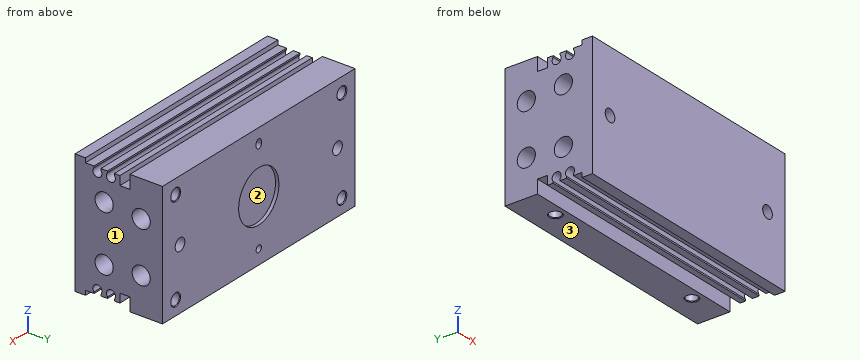
from build123d import *

# Parameters (mm, degrees)
SKETCH2_W                = 55
SKETCH2_H                = 39
BOSS_EXTRUDE1_DEPTH      = 55
CUT_EXTRUDE1_DEPTH       = 65.509689195
CUT_EXTRUDE1_DEPTH_BACK  = 65.509689195
SKETCH3_W                = 2
SKETCH3_H                = 19.8
CUT_EXTRUDE2_DEPTH       = 65.509689195
CUT_EXTRUDE2_DEPTH_BACK  = 65.509689195
SKETCH7_R                = 2.5
CUT_EXTRUDE4_DEPTH       = 10
CHAMFER2_SIZE            = 0.3
SKETCH8_R                = 1.5
CUT_EXTRUDE5_DEPTH       = 3
SKETCH9_R                = 2.75
CUT_EXTRUDE6_DEPTH       = 73.816550317
SKETCH10_R               = 2.5
CUT_EXTRUDE7_DEPTH       = 6
CHAMFER3_SIZE            = 0.3
CUT_EXTRUDE8_DEPTH       = 65.509689195
CUT_EXTRUDE8_DEPTH_BACK  = 65.509689195
SKETCH11_R               = 4.05
SKETCH12_R               = 11.5
CUT_EXTRUDE9_DEPTH       = 1.5
SKETCH13_R               = 5
CUT_EXTRUDE10_DEPTH      = 22.5
CUT_EXTRUDE11_DEPTH      = 65.509689195
CUT_EXTRUDE11_DEPTH_BACK = 65.509689195
SKETCH14_W               = 6
SKETCH14_H               = 4.5


with BuildPart() as part:
    # Sketch2 → Boss-Extrude1 (new, symmetric)
    with BuildSketch(Plane(origin=(0, 0, 0), x_dir=(0, 0, -1), z_dir=(1, 0, 0))):
        Rectangle(SKETCH2_W, SKETCH2_H)
    extrude(amount=BOSS_EXTRUDE1_DEPTH, both=True)

    # Sketch3 → Cut-Extrude1 (cut, two sides: drawn at the far end of the back side and taken through both)
    with BuildSketch(Plane(origin=(0, 0, 0), x_dir=(0, 0, -1), z_dir=(1, 0, 0)).offset(-CUT_EXTRUDE1_DEPTH_BACK)):
        with Locations((-26.5, -4.9)):
            Rectangle(SKETCH3_W, SKETCH3_H)
        with Locations((26.5, -4.9)):
            Rectangle(SKETCH3_W, SKETCH3_H)
    extrude(amount=CUT_EXTRUDE1_DEPTH + CUT_EXTRUDE1_DEPTH_BACK, mode=Mode.SUBTRACT)

    # Sketch5 → Cut-Extrude2 (cut, two sides: drawn at the far end of the back side and taken through both)
    with BuildSketch(Plane(origin=(0, 0, 0), x_dir=(0, 0, -1), z_dir=(1, 0, 0)).offset(-CUT_EXTRUDE2_DEPTH_BACK)):
        with BuildLine():
            Line((-24.822875656, -2), (-25.5, -2))
            Line((-25.5, -2), (-25.5, -5))
            Line((-25.5, -5), (-24.822875656, -5))
            ThreePointArc((-24.822875656, -5), (-21.5, -3.5), (-24.822875656, -2))
        make_face()
        with BuildLine():
            Line((-24.822875656, -8), (-25.5, -8))
            Line((-25.5, -8), (-25.5, -11))
            Line((-25.5, -11), (-24.822875656, -11))
            ThreePointArc((-24.822875656, -11), (-21.5, -9.5), (-24.822875656, -8))
        make_face()
        with BuildLine():
            Line((25.5, -8), (25.5, -11))
            Line((25.5, -11), (24.822875656, -11))
            ThreePointArc((24.822875656, -11), (21.5, -9.5), (24.822875656, -8))
            Line((24.822875656, -8), (25.5, -8))
        make_face()
        with BuildLine():
            Line((25.5, -2), (25.5, -5))
            Line((25.5, -5), (24.822875656, -5))
            ThreePointArc((24.822875656, -5), (21.5, -3.5), (24.822875656, -2))
            Line((24.822875656, -2), (25.5, -2))
        make_face()
    extrude(amount=CUT_EXTRUDE2_DEPTH + CUT_EXTRUDE2_DEPTH_BACK, mode=Mode.SUBTRACT)

    # Sketch7 → Cut-Extrude4 (cut)
    with BuildSketch(Plane(origin=(0, 19.5, 0), x_dir=(1, 0, 0), z_dir=(0, 1, 0))):
        with Locations(Location((-47.5, 21, 0), (0, 0, 270))):
            Circle(SKETCH7_R)
        with Locations(Location((47.5, 21, 0), (0, 0, 270))):
            Circle(SKETCH7_R)
        with Locations(Location((47.5, -21, 0), (0, 0, 270))):
            Circle(SKETCH7_R)
        with Locations(Location((-47.5, -21, 0), (0, 0, 270))):
            Circle(SKETCH7_R)
    extrude(amount=-CUT_EXTRUDE4_DEPTH, mode=Mode.SUBTRACT)

    # Chamfer2
    chamfer2_edges = [part.edges().sort_by_distance(p)[0] for p in [
        (-47.5, 19.5, 18.5),
        (47.5, 19.5, 18.5),
        (47.5, 19.5, -23.5),
        (-47.5, 19.5, -23.5),
    ]]
    chamfer(chamfer2_edges, length=CHAMFER2_SIZE)

    # Sketch8 → Cut-Extrude5 (cut)
    with BuildSketch(Plane(origin=(0, 19.5, 0), x_dir=(1, 0, 0), z_dir=(0, 1, 0))):
        with Locations(Location((0, 21, 0), (0, 0, 270))):
            Circle(SKETCH8_R)
        with BuildLine():
            Line((-1.5, -21.5), (-1.5, -20.5))
            ThreePointArc((-1.5, -20.5), (0, -19), (1.5, -20.5))
            Line((1.5, -20.5), (1.5, -21.5))
            ThreePointArc((1.5, -21.5), (0, -23), (-1.5, -21.5))
        make_face()
    extrude(amount=-CUT_EXTRUDE5_DEPTH, mode=Mode.SUBTRACT)

    # Sketch9 → Cut-Extrude6 (cut, through all)
    with BuildSketch(Plane(origin=(0, 19.5, 0), x_dir=(1, 0, 0), z_dir=(0, 1, 0))):
        with Locations(Location((-45, 0, 0), (0, 0, 270))):
            Circle(SKETCH9_R)
        with Locations(Location((45, 0, 0), (0, 0, 270))):
            Circle(SKETCH9_R)
    extrude(amount=-CUT_EXTRUDE6_DEPTH, mode=Mode.SUBTRACT)

    # Sketch10 → Cut-Extrude7 (cut)
    with BuildSketch(Plane(origin=(0, 0, -27.5), x_dir=(-1, 0, 0), z_dir=(0, 0, -1))):
        with Locations(Location((-39, 9.5, 0), (0, 0, 90))):
            Circle(SKETCH10_R)
        with Locations(Location((39, 9.5, 0), (0, 0, 90))):
            Circle(SKETCH10_R)
    extrude(amount=-CUT_EXTRUDE7_DEPTH, mode=Mode.SUBTRACT)

    # Chamfer3
    chamfer3_edges = [part.edges().sort_by_distance(p)[0] for p in [
        (39, 7, -27.5),
        (-39, 7, -27.5),
    ]]
    chamfer(chamfer3_edges, length=CHAMFER3_SIZE)

    # Sketch11 → Cut-Extrude8 (cut, two sides: drawn at the far end of the back side and taken through both)
    with BuildSketch(Plane(origin=(0, 0, 0), x_dir=(0, 0, -1), z_dir=(1, 0, 0)).offset(-CUT_EXTRUDE8_DEPTH_BACK)):
        with Locations((-11.3, 10)):
            Circle(SKETCH11_R)
        with Locations((11.3, 10)):
            Circle(SKETCH11_R)
        with Locations((-12.5, -6.5)):
            Circle(SKETCH11_R)
        with Locations((12.5, -6.5)):
            Circle(SKETCH11_R)
    extrude(amount=CUT_EXTRUDE8_DEPTH + CUT_EXTRUDE8_DEPTH_BACK, mode=Mode.SUBTRACT)

    # Sketch12 → Cut-Extrude9 (cut)
    with BuildSketch(Plane(origin=(0, 19.5, 0), x_dir=(1, 0, 0), z_dir=(0, 1, 0))):
        with Locations(Location((0, 0, 0), (0, 0, 270))):
            Circle(SKETCH12_R)
    extrude(amount=-CUT_EXTRUDE9_DEPTH, mode=Mode.SUBTRACT)

    # Sketch13 → Cut-Extrude10 (cut, symmetric)
    with BuildSketch(Plane(origin=(0, 0, 0), x_dir=(0, 0, -1), z_dir=(1, 0, 0))):
        with Locations((-11.3, 10)):
            Circle(SKETCH13_R)
        with Locations((11.3, 10)):
            Circle(SKETCH13_R)
        with Locations((12.5, -6.5)):
            Circle(SKETCH13_R)
        with Locations((-12.5, -6.5)):
            Circle(SKETCH13_R)
    extrude(amount=CUT_EXTRUDE10_DEPTH, both=True, mode=Mode.SUBTRACT)

    # Sketch14 → Cut-Extrude11 (cut, two sides: drawn at the far end of the back side and taken through both)
    with BuildSketch(Plane(origin=(0, 0, 0), x_dir=(0, 0, -1), z_dir=(1, 0, 0)).offset(-CUT_EXTRUDE11_DEPTH_BACK)):
        with Locations((-24.5, 2.75)):
            Rectangle(SKETCH14_W, SKETCH14_H)
        with Locations((24.5, 2.75)):
            Rectangle(SKETCH14_W, SKETCH14_H)
    extrude(amount=CUT_EXTRUDE11_DEPTH + CUT_EXTRUDE11_DEPTH_BACK, mode=Mode.SUBTRACT)


solid = part.part
Can you work these out from the model? Positions are in its coordinate system, mm. Face numbers are marked on the shaded views. Give positions to 0.01 mm unless a question says otherwise; leave off trailing zeros. Write each loop counter-clockwise with the first axis right and the second up, starting at its lowest first coordinate (ties: lowest second). Pieces come first, ordered by that corner, then holes. Notation, with made-up numbers: M -34,51 L 7,51 A20 ccw 7,89 Z; hole C 61,-36.75 d3. An arc over 180 degrees is marked long. Answer in a Markdown table with one row per item. Add a question column.
Item 1: For pin 1 Ø2 at (x, y) = (-22, -0.5) entering from +Z; pin 2 Ø8 at (y, z) = (-6.5, 12.5) entering from -X; pin 3 Ø1.5 at (x, z) = (46.5, -20) entering from +Y; pin 4 Ø3.5 at (x, y) = (5, -7) entering from -Z, each with a flat end and sliding along its axis, tell me the tip position at first contact or that it passes through.
Item 2: We'd pull the mould along Z, two halves only. Please class the marked faces 1, 2 and 3: released by +Z, released by -Z, zero draft, split by the parting line, or undercut.
Item 3: Imagine slicing it at D-D, the plane z = 13.5. Write out the boundary of the cut face in (x, y), plus the area to 3 significant figures.
Item 4: Please list where these lines run through material, in increasing order: L1, parallel to Z at x = -1, y = -6; L2, parallel to Z at x = 38, y = 10; L3, parallel to Y at x = 24.5, z = -24.
Item 5: Imagine slicing it at A-A, the plane z = 0. Write out the boundary of the cut face in (x, y).
Item 6: Imagine slicing it at B-B, the plane y = -3.5. State how many separate pieces and enclosed holes the cut face has, plus the area to 3 significant figures.
Evaluation:
| question | item | result |
|---|---|---|
| 1 | pin 1 | stops at z = 25.5 |
| 1 | pin 2 | passes through |
| 1 | pin 3 | stops at y = 9.5 |
| 1 | pin 4 | stops at z = -25.5 |
| 2 | face 1 | zero draft |
| 2 | face 2 | undercut |
| 2 | face 3 | released by -Z |
| 3 | outline | M -55,-19.5 L 55,-19.5 L 55,-10.42 L 22.5,-10.42 L 22.5,-11.4 L -22.5,-11.4 L -22.5,-10.42 L -55,-10.42 Z; M -55,-2.58 L -22.5,-2.58 L -22.5,-1.6 L 22.5,-1.6 L 22.5,-2.58 L 55,-2.58 L 55,6.6 L 22.5,6.6 L 22.5,5.51 L -22.5,5.51 L -22.5,6.6 L -55,6.6 Z; M -55,13.4 L -22.5,13.4 L -22.5,14.49 L 22.5,14.49 L 22.5,13.4 L 55,13.4 L 55,19.5 L -55,19.5 Z |
| 3 | area | 2,490 mm² |
| 4 | L1 | z = -25.5 to -17.47, -7.53 to 7.53, 17.47 to 25.5 |
| 4 | L2 | z = -21.5 to -15.35, -7.25 to 7.25, 15.35 to 27.5 |
| 4 | L3 | y = -19.5 to -11.44, -7.56 to -5.44, -1.56 to 0.5, 5 to 19.5 |
| 5 | outline | M -55,-19.5 L -47.75,-19.5 L -47.75,19.5 L -55,19.5 Z; M -42.25,-19.5 L 42.25,-19.5 L 42.25,19.5 L 11.5,19.5 L 11.5,18 L -11.5,18 L -11.5,19.5 L -42.25,19.5 Z; M 47.75,-19.5 L 55,-19.5 L 55,19.5 L 47.75,19.5 Z |
| 6 | separate pieces | 3 |
| 6 | enclosed holes | 2 |
| 6 | area | 3,260 mm² |
